Geometry check sheet. Reference: the model listing, model coordinates, mm. A direction names the side the tool comes from. Coordinates: 2 decimals unless noted, no trailing zeros. Loops run counter-clockwise (first coordinate to the right, second up) from the corner with the lowest first, then second, coordinate; pieces in that order, holes last. Notation, with made-up numbers: (76, 38.25) - (100, 38.25) arc R20 ccw to (100, 72.25) - close; hole circle Ø2 at (3.5, 32). An arc over 180 degrees is marked (long way). Write each question's results on one line, items separated by ' | '. Start each with the question number.
(1) Go/stop test with flat-tipped pins: pin 1 Ø3 at (x, y) = (-4, -19) entering from +Z; pin 2 Ø10 at (x, z) = (-19, 19) entering from +Y; pin 3 Ø10 at (x, z) = (19, 20.5) entering from -Y. Record where each tip stops, or that it passes through.
(2) Sectioned sample at A-A (y = 18). Enter the section's corners in (x, z).
(3) Access from +Z, -Z, +X, -X, +Y, -Y to the whole of each face (thin tool, end or side, straight path). Record for faces 1 (the face through (-1, 3.5, 20)), 2 (the face through (-44, 12, 3)), 3 (the face through (-1, -3.5, 20)).
(4) Sectioned sample at D-D (z = 7). Enter the section's corners in (x, y).
(5) Sectioned sample at C-C (y = -21). Enter the section's corners in (x, z).
(6) Mould release check, pull along Y, two halves, no side actions. Record for faces 4 (the face through (-45, -15, 3)), 5 (the face through (-47.15, -21.99, 2.54)), 6 (the face through (-47.15, 21.99, 2.54)): pulls with the +Y half, pulls with the -Y half, needs draft (parallel to the pull), parting line crosses it, or undercut.
(7) Material ranges on probe 1 along Y at (x, z) = (-40, 1.45); probe 2 along Y at (x, z) = (-24, 23); probe 3 along Z at (x, y) = (30.5, -18.5), recorded low to high.
(8) Sectioned sample at B-B (x = 5). Enter the section's corners in (y, z).
from build123d import *

# Parameters (mm, degrees)
SKETCH_W     = 100
SKETCH_H     = 50
PAD_DEPTH    = 5
SKETCH001_R  = 5
POCKET_DEPTH = 5
SKETCH002_W  = 100
SKETCH002_H  = 7
PAD001_DEPTH = 25
FILLET_R     = 20
FILLET001_R  = 10
FILLET002_R  = 5


with BuildPart() as part:
    # Sketch → Pad (new body)
    with BuildSketch(Plane.XY):
        Rectangle(SKETCH_W, SKETCH_H)
    extrude(amount=PAD_DEPTH)

    # Sketch001 (on Face6 of Pad) → Pocket (cut)
    with BuildSketch(Plane.XY.offset(5)):
        with Locations((-40, 15)):
            Circle(SKETCH001_R)
        with Locations((40, 15)):
            Circle(SKETCH001_R)
        with Locations((40, -15)):
            Circle(SKETCH001_R)
        with Locations((-40, -15)):
            Circle(SKETCH001_R)
    extrude(amount=-POCKET_DEPTH, mode=Mode.SUBTRACT)

    # Sketch002 (on Face5 of Pocket) → Pad001 (join)
    with BuildSketch(Plane.XY.offset(5)):
        Rectangle(SKETCH002_W, SKETCH002_H)
    extrude(amount=PAD001_DEPTH)

    # Fillet
    fillet_edges = [part.edges().sort_by_distance(p)[0] for p in [
        (-50, 0, 30),
        (50, 0, 30),
    ]]
    fillet(fillet_edges, radius=FILLET_R)

    # Fillet001
    fillet001_edges = [part.edges().sort_by_distance(p)[0] for p in [
        (50, -25, 2.5),
        (-50, -25, 2.5),
        (-50, 25, 2.5),
        (50, 25, 2.5),
    ]]
    fillet(fillet001_edges, radius=FILLET001_R)

    # Fillet002
    fillet002_edges = [part.edges().sort_by_distance(p)[0] for p in [
        (0, -3.5, 5),
        (0, 3.5, 5),
    ]]
    fillet(fillet002_edges, radius=FILLET002_R)


solid = part.part
Outcome:
1) pin 1: stops at z = 5 | pin 2: stops at y = 3.5 | pin 3: stops at y = -3.5
2) outline: (-49.54, 0) - (-44, 0) - (-44, 5) - (-49.54, 5) - close; (-36, 0) - (36, 0) - (36, 5) - (-36, 5) - close; (44, 0) - (49.54, 0) - (49.54, 5) - (44, 5) - close
3) face 1: +Z, +X, -X, +Y | face 2: +Z, -Z | face 3: +Z, +X, -X, -Y
4) outline: (-50, -4.5) - (50, -4.5) - (50, 4.5) - (-50, 4.5) - close
5) outline: (-48, 0) - (48, 0) - (48, 5) - (-48, 5) - close
6) face 4: undercut | face 5: pulls with the -Y half | face 6: pulls with the +Y half
7) probe 1: y = -25 to -20, -10 to 10, 20 to 25 | probe 2: y = -3.5 to 3.5 | probe 3: z = 0 to 5
8) outline: (-25, 0) - (25, 0) - (25, 5) - (8.5, 5) arc R5 cw to (3.5, 10) - (3.5, 30) - (-3.5, 30) - (-3.5, 10) arc R5 cw to (-8.5, 5) - (-25, 5) - close
